from build123d import *

# Parameters (mm, degrees)
F0_R     = 1.575
F0_R_2   = 3.05
F1_DEPTH = 4


with BuildPart() as f1:
    # F0 (on Top) → F1 (new body)
    with BuildSketch(Plane.XY):
        with BuildLine():
            ThreePointArc((-66.362554, 3.889581), (-62.092779, -3.869236), (-56.183578, -10.465566))
            ThreePointArc((-56.183578, -10.465566), (-42.950605, -37.701035), (-17.660321, -54.35288))
            Line((-17.660321, -54.35288), (-22.897159, -60.400651))
            ThreePointArc((-22.897159, -60.400651), (-14.960223, -59.333067), (-7.408336, -56.667796))
            ThreePointArc((-7.408336, -56.667796), (22.583349, -52.498713), (46.235321, -33.591927))
            Line((46.235321, -33.591927), (51.402196, -42.153668))
            ThreePointArc((51.402196, -42.153668), (52.508394, -33.366942), (51.604975, -24.557058))
            ThreePointArc((51.604975, -24.557058), (56.907882, 5.255046), (46.235321, 33.591927))
            Line((46.235321, 33.591927), (55.974673, 35.860194))
            ThreePointArc((55.974673, 35.860194), (47.959834, 39.627498), (39.301964, 41.490699))
            ThreePointArc((39.301964, 41.490699), (12.587657, 55.74651), (-17.660321, 54.35288))
            Line((-17.660321, 54.35288), (-16.807946, 64.316486))
            ThreePointArc((-16.807946, 64.316486), (-22.867587, 57.858083), (-27.315025, 50.19972))
            ThreePointArc((-27.315025, 50.19972), (-49.128282, 29.198192), (-57.15, 0))
            Line((-57.15, 0), (-66.362554, 3.889581))
        make_face()
        with BuildLine():
            ThreePointArc((-33.939505, -34.900173), (-42.205105, -24.367129), (-47.194189, -11.942387))
            ThreePointArc((-47.194189, -11.942387), (-46.760906, -9.079501), (-44.198279, -7.731618))
            Line((-44.198279, -7.731618), (-20.853145, -7.357517))
            ThreePointArc((-20.853145, -7.357517), (-17.06203, -9.850768), (-16.798369, -14.380595))
            Line((-16.798369, -14.380595), (-28.794917, -34.411023))
            ThreePointArc((-28.794917, -34.411023), (-31.243532, -35.956382), (-33.939505, -34.900173))
        make_face(mode=Mode.SUBTRACT)
        with Locations((-10, 0)):
            Circle(F0_R, mode=Mode.SUBTRACT)
        with BuildLine():
            ThreePointArc((13.254683, -46.84256), (0, -48.734257), (-13.254683, -46.84256))
            ThreePointArc((-13.254683, -46.84256), (-15.517374, -45.035883), (-15.403362, -42.142641))
            Line((-15.403362, -42.142641), (-4.054776, -21.738112))
            ThreePointArc((-4.054776, -21.738112), (0, -19.701535), (4.054776, -21.738112))
            Line((4.054776, -21.738112), (15.403362, -42.142641))
            ThreePointArc((15.403362, -42.142641), (15.517374, -45.035883), (13.254683, -46.84256))
        make_face(mode=Mode.SUBTRACT)
        with Locations((0, -10)):
            Circle(F0_R, mode=Mode.SUBTRACT)
        Circle(F0_R_2, mode=Mode.SUBTRACT)
        with Locations((10, 0)):
            Circle(F0_R, mode=Mode.SUBTRACT)
        with BuildLine():
            ThreePointArc((47.194189, -11.942387), (42.205105, -24.367129), (33.939505, -34.900173))
            ThreePointArc((33.939505, -34.900173), (31.243532, -35.956382), (28.794917, -34.411023))
            Line((28.794917, -34.411023), (16.798369, -14.380595))
            ThreePointArc((16.798369, -14.380595), (17.06203, -9.850768), (20.853145, -7.357517))
            Line((20.853145, -7.357517), (44.198279, -7.731618))
            ThreePointArc((44.198279, -7.731618), (46.760906, -9.079501), (47.194189, -11.942387))
        make_face(mode=Mode.SUBTRACT)
        with BuildLine():
            ThreePointArc((-47.194189, 11.942387), (-42.205105, 24.367129), (-33.939505, 34.900173))
            ThreePointArc((-33.939505, 34.900173), (-31.243532, 35.956382), (-28.794917, 34.411023))
            Line((-28.794917, 34.411023), (-16.798369, 14.380595))
            ThreePointArc((-16.798369, 14.380595), (-17.06203, 9.850768), (-20.853145, 7.357517))
            Line((-20.853145, 7.357517), (-44.198279, 7.731618))
            ThreePointArc((-44.198279, 7.731618), (-46.760906, 9.079501), (-47.194189, 11.942387))
        make_face(mode=Mode.SUBTRACT)
        with Locations((0, 10)):
            Circle(F0_R, mode=Mode.SUBTRACT)
        with BuildLine():
            ThreePointArc((20.853145, 7.357517), (17.06203, 9.850768), (16.798369, 14.380595))
            Line((16.798369, 14.380595), (28.794917, 34.411023))
            ThreePointArc((28.794917, 34.411023), (31.243532, 35.956382), (33.939505, 34.900173))
            ThreePointArc((33.939505, 34.900173), (42.205105, 24.367129), (47.194189, 11.942387))
            ThreePointArc((47.194189, 11.942387), (46.760906, 9.079501), (44.198279, 7.731618))
            Line((44.198279, 7.731618), (20.853145, 7.357517))
        make_face(mode=Mode.SUBTRACT)
        with BuildLine():
            Line((15.403362, 42.142641), (4.054776, 21.738112))
            ThreePointArc((4.054776, 21.738112), (0, 19.701535), (-4.054776, 21.738112))
            Line((-4.054776, 21.738112), (-15.403362, 42.142641))
            ThreePointArc((-15.403362, 42.142641), (-15.517374, 45.035883), (-13.254683, 46.84256))
            ThreePointArc((-13.254683, 46.84256), (0, 48.734257), (13.254683, 46.84256))
            ThreePointArc((13.254683, 46.84256), (15.517374, 45.035883), (15.403362, 42.142641))
        make_face(mode=Mode.SUBTRACT)
    extrude(amount=F1_DEPTH)


solid = f1.part
Could you check a few things on this model? Use its own coordinates, in mm. Give positions to 0.01 mm unless a question says otherwise; leave off trailing zeros. Order: outer loops, then holes, each group sorted by start corner. A loop starts at its lowest first (then second) coordinate and runs counter-clockwise, first axis right, second up. Notation, with made-up numbers: (-22.5, -7) - (-12.5, -7) arc R19 ccw to (-12.5, 29) - close; hole circle Ø3 at (-2, 79). An arc over 180 degrees is marked (long way). One line per question, with ' | ' between items. Start each with the question number.
Item 1: I want a section at A-A on x = 0. Write out the boundary of the cut face in (y, z) (3 decimals), then the cut area to 3 significant figures.
Item 2: I need wall thicknesses on probe 1 along Y at (x, z) = (0, 3.1) (3 decimals); probe 2 along Y at (x, z) = (40, 1.45); probe 3 along Y at (x, z) = (2, 2.9) (3 decimals). Which ranges of each line are inside material? Lowest first, please. Write a range as [from, to].
Item 3: Thinking about a two-plate mould opening in X: for faces 1 (the cylindrical face through (-11.573, 0.069, 1.972)), 2 (the flat face through (-20.24, -57.33, 1.97)), 3 (the flat face through (8, 3, 4)), which applies, pulls with the +X half, pulls with the -X half, needs draft (parallel to the pull), parting line crosses it, or undercut?
Item 4: I'm going to push flat-ended pins straight in: pin 1 Ø1 at (y, z) = (-32.5, 3) entering from +X; pin 2 Ø4 at (x, y) = (0, 10) entering from +Z; pin 3 Ø1.5 at (x, z) = (-33.5, 3) entering from -Y; pin 4 Ø1.5 at (x, z) = (40, 3) entering from -Y. Where does each tip first touch, or does it pass through?
Item 5: I want a section at D-D on y = -39. Write out the boundary of the cut face in (x, z).
Item 6: I want a section at C-C on x = 41.5. Write out the boundary of the cut face in (y, z).
Item 7: I want a section at B-B on y = 24. Write out the boundary of the cut face in (x, z), then the cut area to 3 significant figures.
Verdict:
1) outline: (-57.15, 0) - (-48.734, 0) - (-48.734, 4) - (-57.15, 4) - close; (-19.702, 0) - (-11.575, 0) - (-11.575, 4) - (-19.702, 4) - close; (-8.425, 0) - (-3.05, 0) - (-3.05, 4) - (-8.425, 4) - close; (3.05, 0) - (8.425, 0) - (8.425, 4) - (3.05, 4) - close; (11.575, 0) - (19.702, 0) - (19.702, 4) - (11.575, 4) - close; (48.734, 0) - (57.15, 0) - (57.15, 4) - (48.734, 4) - close | area: 175 mm^2
2) probe 1: [-57.15, -48.734], [-19.702, -11.575], [-8.425, -3.05], [3.05, 8.425], [11.575, 19.702], [48.734, 57.15] | probe 2: [-40.82, -27.83], [-7.66, 7.66], [27.83, 41.42] | probe 3: [-57.115, -48.692], [-20.114, -2.303], [2.303, 20.114], [48.692, 57.115]
3) face 1: undercut | face 2: pulls with the -X half | face 3: needs draft
4) pin 1: x = 52.51 | pin 2: z = 4 | pin 3: y = -46.84 | pin 4: y = -41.54
5) outline: (-41.77, 0) - (-13.66, 0) - (-13.66, 4) - (-41.77, 4) - close; (13.66, 0) - (41.77, 0) - (41.77, 4) - (13.66, 4) - close; (49.5, 0) - (52.03, 0) - (52.03, 4) - (49.5, 4) - close
6) outline: (-39.29, 0) - (-25.55, 0) - (-25.55, 4) - (-39.29, 4) - close; (-7.69, 0) - (7.69, 0) - (7.69, 4) - (-7.69, 4) - close; (25.55, 0) - (41.21, 0) - (41.21, 4) - (25.55, 4) - close
7) outline: (-51.87, 0) - (-42.41, 0) - (-42.41, 4) - (-51.87, 4) - close; (-22.56, 0) - (-5.31, 0) - (-5.31, 4) - (-22.56, 4) - close; (5.31, 0) - (22.56, 0) - (22.56, 4) - (5.31, 4) - close; (42.41, 0) - (51.87, 0) - (51.87, 4) - (42.41, 4) - close | area: 214 mm^2
